from build123d import *

# Parameters (mm, degrees)
F2_W     = 13.42322
F2_H     = 3.613965
F3_DEPTH = 12.5


with BuildPart() as f1:
    # F0 (on Front) → F1 (revolve)
    with BuildSketch(Plane.XZ):
        Polygon((2.658645, 4), (0, 0), (50, 0), (50, 12.5), (25.722432, 12.5), (11, 4), align=None)
    revolve(axis=Axis((25, 0, 0), (-1, 0, 0)))

    # F2 (on Front) → F3 (cut, symmetric)
    with BuildSketch(Plane.XZ):
        with Locations((46.71161, 13.306983)):
            Rectangle(F2_W, F2_H)
        with Locations((46.71161, -13.306983)):
            Rectangle(F2_W, F2_H)
    extrude(amount=F3_DEPTH, both=True, mode=Mode.SUBTRACT)


solid = f1.part
Can you work these out from the model? Positions are in its coordinate system, mm. A direction names the side the tool comes from. Round coordinates to 2 decimals unless told otherwise and drop trailing zeros. Write each loop counter-clockwise with the first axis right and the second up, starting at its lowest first coordinate (ties: lowest second). Pieces come first, ordered by that corner, then holes. Notation, with made-up numbers: (-36, -8) -> (-29, -8) arc R12 ccw to (-29, 15) -> close; hole circle Ø7 at (79.25, -15.75). An arc over 180 degrees is marked (long way). One line per question, with ' | ' between items. Start each with the question number.
1) Suppose I cut it at B-B on x = 43. Write out the boundary of the cut face in (y, z), then the cut area to 3 significant figures.
2) I need wall thicknesses on line 1 (Z direction, x = 44, y = -0.5); line 2 (Z direction, x = 43, y = -10); line 3 (X direction, y = -4, z = 3.5). Which ranges of each line are inside material? Lowest first, please. Write a range as [from, to].
3) Suppose I cut it at A-A on x = 30. Write out the boundary of the cut face in (y, z), then the cut area to 3 significant figures.
4) Suppose I cut it at C-C on x = 17.5. Write out the boundary of the cut face in (y, z).
5) I'm going to push flat-ended pins straight in: P1, Ø3, axis at x = 43, y = -2, coming from the -Z side; P2, Ø8, axis at y = -0.5, z = 6.5, coming from the -X side; P3, Ø8, axis at x = 10, z = -1.5, coming from the +Y side; P4, Ø6, axis at x = 25, y = -0.5, coming from the +Z side. Where does each tip first touch, or does it pass through?
6) On a 3-axis mill with a long thin cutter (end or side, diameter ignored), from which of +Z, -Z, +X, -X, +Y, -Y can I reach the whole of each face in a straight line? I mean faces 1 (the flat face through (45, 0, 11.5)), 2 (the cylindrical face through (6.771, -3.905, -0.867)), 3 (the flat face through (40, 0, -12)), 4 (the cylindrical face through (37.691, 0.55, -12.488)), 5 (the flat face through (50, 0, 0)). Say none if no direction works.
Return value:
1) outline: (-4.9, -11.5) -> (4.9, -11.5) arc R12.5 ccw to (4.9, 11.5) -> (-4.9, 11.5) arc R12.5 ccw to start | area: 478 mm2
2) line 1: z = [-11.5, 11.5] | line 2: z = [-7.5, 7.5] | line 3: x = [13.28, 50]
3) outline: circle Ø25 at (0, 0) | area: 491 mm2
4) outline: circle Ø15.51 at (0, 0)
5) P1: stops at z = -11.5 | P2: stops at x = 1.67 | P3: stops at y = 5.64 | P4: stops at z = 12.5
6) face 1: +Z, +X, +Y, -Y | face 2: -X | face 3: -Z, +X, +Y, -Y | face 4: +X, -X | face 5: +Z, -Z, +X, +Y, -Y
